CAD build for the part. Positions are in the model's coordinates, mm. Face numbers are marked on the shaded views. A direction names the side the tool comes from. Round coordinates to 2 decimals unless told otherwise and drop trailing zeros. Order: outer loops, then holes, each group sorted by start corner. A loop starts at its lowest first (then second) coordinate and runs counter-clockwise, first axis right, second up. Notation, with made-up numbers: M 1.5,73 L 30.5,73 A20 cw 30.5,96 Z; hole C 16.5,55 d5. An arc over 180 degrees is marked long. Answer as a JSON object with one key per item and string values. Group by question number.
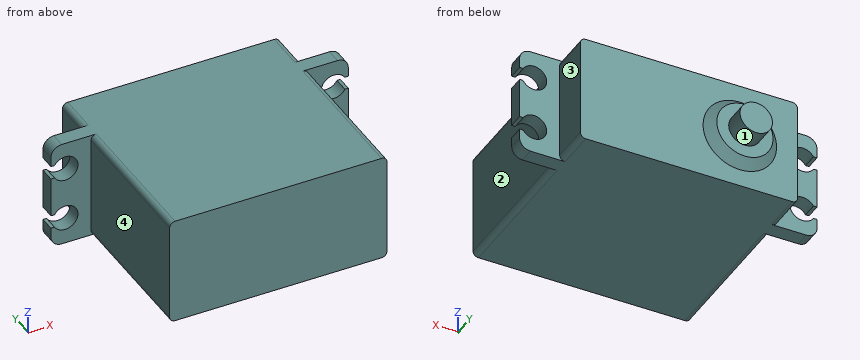
Autodesk Inventor part; units mm, degrees
ref_plane "YZ Plane" through (0, 0, 0) normal (1, 0, 0) x (0, 1, 0)
ref_plane "XZ Plane" through (0, 0, 0) normal (0, 1, 0) x (-1, 0, 0)
ref_plane "XY Plane" through (0, 0, 0) normal (0, 0, 1) x (1, 0, 0)
sketch "Sketch1" plane through (0, 0, 0) normal (0, 1, 0) x (-1, 0, 0)
  line L0 (-20.1, -10) -> (20.1, -10)
  line L1 (20.1, -10) -> (20.1, 10)
  line L2 (20.1, 10) -> (-20.1, 10)
  line L3 (-20.1, 10) -> (-20.1, -10)
  line L4 (-20.1, -10) -> (20.1, 10) construction
  line L5 (20.1, -10) -> (-20.1, 10) construction
  point P0 (0, 0)
extrude "Extrusion1" add sketch "Sketch1" along normal blind 43.7
sketch "Sketch2" plane through (20.1, 0, 10) normal (1, 0, 0) x (0, 0, -1)
  line L0 (20, 0) -> (20, 43.7)
  line L1 (0, 0) -> (0, 43.7)
  line L2 (20, 27.8) -> (0, 27.8)
  line L3 (0, 27.8) -> (0, 30.6)
  line L4 (0, 30.6) -> (20, 30.6)
  line L5 (20, 30.6) -> (20, 27.8)
  point P0 (10, 0)
sketch "Sketch3" plane through (-20.1, 0, -10) normal (-1, 0, 0) x (0, 0, 1)
  line L0 (20, 0) -> (20, 43.7)
  line L1 (0, 0) -> (0, 43.7)
  line L2 (20, 27.8) -> (0, 27.8)
  line L3 (0, 27.8) -> (0, 30.6)
  line L4 (0, 30.6) -> (20, 30.6)
  line L5 (20, 30.6) -> (20, 27.8)
  point P0 (10, 0)
extrude "Extrusion2" add sketch "Sketch3" along normal blind 7.4
extrude "Extrusion3" add sketch "Sketch2" along normal blind 7.4
sketch "Sketch4" plane through (0, 43.7, 0) normal (0, 1, 0) x (1, 0, 0)
  line L0 (20.1, 10) -> (-20.1, 10)
  line L1 (-20.1, 10) -> (-20.1, -10)
  line L2 (-20.1, -10) -> (20.1, -10)
  line L3 (20.1, -10) -> (20.1, 10)
  circle A0 centre (-9.4, 0) radius 6.8
  circle A1 centre (-9.4, 0) radius 5.1
  circle A2 centre (-9.4, 0) radius 3
extrude "Extrusion4" cut sketch "Sketch4" against normal blind 5.8 contours L3 L2 L1 L0
sketch "Sketch5" plane through (-9.4, 43.7, 0) normal (0, 1, 0) x (1, 0, 0)
  circle A0 centre (0, 0) radius 6.8
  circle A1 centre (0, 0) radius 2.5
  dimension "d20" = 5
extrude "Extrusion5" cut sketch "Sketch5" against normal blind 4
fillet "Fillet1" radius 2 1 edges at (-27.5, 29.2, 10)
fillet "Fillet2" radius 2 1 edges at (27.5, 29.2, 10)
fillet "Fillet3" radius 2 1 edges at (27.5, 29.2, -10)
fillet "Fillet4" radius 2 1 edges at (-27.5, 29.2, -10)
fillet "Fillet5" radius 1 1 edges at (-20.1, 34.25, -10)
fillet "Fillet6" radius 1 1 edges at (-20.1, 13.9, -10)
fillet "Fillet7" radius 1 1 edges at (-20.1, 34.25, 10)
fillet "Fillet8" radius 1 1 edges at (-20.1, 13.9, 10)
fillet "Fillet9" radius 1 1 edges at (20.1, 34.25, 10)
fillet "Fillet10" radius 1 1 edges at (20.1, 13.9, 10)
fillet "Fillet11" radius 1 1 edges at (20.1, 34.25, -10)
fillet "Fillet12" radius 1 1 edges at (20.1, 13.9, -10)
sketch "Sketch6" plane through (-9.4, 43.7, 0) normal (0, 1, 0) x (1, 0, 0)
  circle A0 centre (0, 0) radius 3
  point P0 (9.4, 0)
extrude "Extrusion6" add sketch "Sketch6" against normal blind 4
chamfer "Chamfer3" distance 1.8 distance2 1.6 1 edges at (-16.2, 39.7, 0) measured on face at (-2.6881, 38.5, 1.0908)
sketch "Sketch7" plane through (27.5, 30.6, 8) normal (0, 1, 0) x (1, 0, 0)
  circle A0 centre (-2.65, 12.95) radius 2.35
  circle A1 centre (-2.65, 3.05) radius 2.35
  line L0 (-0.0003, 1.8) -> (-0.66, 1.8)
  line L1 (-0.0003, 4.222) -> (-0.6131, 4.222)
  line L2 (-0.0003, 12.95) -> (-0.0003, 14.2)
  line L3 (-0.0003, 14.2) -> (-0.66, 14.2)
  line L4 (-0.0003, 12.95) -> (-0.0003, 11.7)
  line L5 (-0.0003, 11.7) -> (-0.66, 11.7)
  line L6 (-0.0003, 4.222) -> (-0.0003, 1.8)
  line L7 (0, 16) -> (0, 0)
  line L8 (-0.0003, 14.2) -> (2.6929, 14.2)
  line L9 (-0.0003, 11.7) -> (2.6929, 11.7)
  line L10 (2.6929, 11.7) -> (2.6929, 14.2)
  line L11 (-0.0003, 4.222) -> (2.459, 4.222)
  line L12 (-0.0003, 1.8) -> (2.459, 1.8)
  line L13 (2.459, 1.8) -> (2.459, 4.222)
  point P0 (-27.5, 8)
sketch "Sketch8" plane through (-27.5, 30.6, 8) normal (0, 1, 0) x (1, 0, 0)
  circle A0 centre (2.65, 12.95) radius 2.35
  circle A1 centre (2.65, 3.05) radius 2.35
  line L0 (0, 3.05) -> (0, 4.3)
  line L1 (0, 4.3) -> (0, 1.8)
  line L2 (0, 4.3) -> (0.66, 4.3)
  line L3 (0, 1.8) -> (0.66, 1.8)
  line L4 (0, 12.95) -> (0, 11.7)
  line L5 (0, 11.7) -> (0.66, 11.7)
  line L6 (0, 12.95) -> (0, 14.2)
  line L7 (0, 14.2) -> (0.66, 14.2)
  point P0 (27.5, 8)
extrude "Extrusion7" cut sketch "Sketch7" against normal blind 3
extrude "Extrusion8" cut sketch "Sketch8" against normal blind 3
properties part number "standart_servo"
Item 1: Cut at B-B, the plane y = 3. Give the cut face in (x, z), and give its area (3 significant figures).
Item 2: Cut at D-D, the plane x = 0. Give the cut face in (y, z), and give its area (3 significant figures).
Item 3: Flat gauge pins, fed straight in: pin 1 Ø1.5 at (x, z) = (-8, 6.5) entering from +Y; pin 2 Ø2 at (y, z) = (34.5, -3.5) entering from -X; pin 3 Ø4 at (x, z) = (-22, -0.5) entering from +Y; pin 4 Ø4 at (x, z) = (24.85, -4.95) entering from +Y. Where does each tip first touch, or does it go through?
Item 4: Cut at A-A, the plane x = -24.85. Give the cut face in (y, z).
Item 5: Drill centre lines: line 1 (Z direction, x = -24.85, y = 29.65); line 2 (X direction, y = 30.5, z = 6.5); line 3 (X direction, y = 29, z = 3.25). Where is each one in solid material? Low to high. Write a range as [from, to].
Item 6: 3-axis set-ups, long thin cutter, end or side, ignore diameter. For the marked faces 1, 2, 3 and 4: which of +Z, -Z, +X, -X, +Y, -Y reach the whole face in a straight line?
Response values:
{
 "1": {"outline": "M -20.1,-9 A1 ccw -19.1,-10 L 19.1,-10 A1 ccw 20.1,-9 L 20.1,9 A1 ccw 19.1,10 L -19.1,10 A1 ccw -20.1,9 Z", "area": "803 mm^2"},
 "2": {"outline": "M 0,-10 L 37.9,-10 L 37.9,10 L 0,10 Z", "area": "758 mm^2"},
 "3": {"pin 1": "y = 38.91", "pin 2": "x = -20.1", "pin 3": "y = 37.9", "pin 4": "through"},
 "4": {"outline": "M 27.8,-10 L 30.6,-10 L 30.6,-7.3 L 27.8,-7.3 Z; M 27.8,-2.6 L 30.6,-2.6 L 30.6,2.6 L 27.8,2.6 Z; M 27.8,7.3 L 30.6,7.3 L 30.6,10 L 27.8,10 Z"},
 "5": {"line 1": "[-10, -7.3], [-2.6, 2.6], [7.3, 10]", "line 2": "[-27.5, -26.62], [-23.08, 23.08], [26.62, 27.5]", "line 3": "[-27.5, -26.47], [-23.23, 23.23], [26.47, 27.5]"},
 "6": {"face 1": "+Y", "face 2": "+Z, -Z, +X, -Y", "face 3": "+Z, -Z, +X, +Y", "face 4": "+Z, -Z, -X, -Y"}
}
